Autodesk Fusion 360 part; units mm, degrees
sketch "Sketch1" plane through (0, 0, 0) normal (0, 0, 1) x (1, 0, 0)
  line L0 (0, -25) -> (-80, 0)
  line L1 (-80, 0) -> (0, 25)
  line L2 (80, 0) -> (0, 25)
  line L3 (80, 0) -> (0, -25)
extrude "Extrude1" add sketch "Sketch1" along normal blind 10 makes body 1
fillet "Fillet3" radius 20 1 edges at (0, 25, 5) on bodies 1
fillet "Fillet4" radius 20 1 edges at (0, -25, 5) on bodies 1
sketch "Sketch5" plane through (0, 0, 10) normal (0, 0, 1) x (-1, 0, 0)
  arc A0 (5.9655, 23.1358) -> (-5.9655, 23.1358) centre (0, 4.0462) ccw
  line L0 (-5.9655, 23.1358) -> (-80, 0)
  line L1 (-80, 0) -> (-5.9655, -23.1358)
  arc A1 (-5.9655, -23.1358) -> (5.9655, -23.1358) centre (0, -4.0462) ccw
  line L2 (5.9655, -23.1358) -> (80, 0)
  line L3 (80, 0) -> (5.9655, 23.1358)
  circle A2 centre (0, 0) radius 20
  circle A3 centre (0, 0) radius 12.5
  dimension "d19" = 25
extrude "Extrude5" add sketch "Sketch5" along normal blind 25 contours A2 bodies 1
extrude "Extrude6" cut 1 faces at (-0.8448, -2.1525, 10) along direction (0, 0, -1) blind 60 on bodies 1 bodies 1
sketch "Sketch8" plane through (0, 0, 0) normal (0, 1, 0) x (1, 0, 0)
  line L0 (-20, -30) -> (-30, -10)
  line L1 (-30, -10) -> (-20, -10)
  line L2 (-20, -10) -> (-20, -30)
  line L3 (20, -30) -> (30, -10)
  line L4 (30, -10) -> (20, -10)
  line L5 (20, -10) -> (20, -30)
extrude "Extrude8" add sketch "Sketch8" along normal blind 2.5 separate body makes body 2 at (-23.3333, 0, 16.6667) makes body 3 at (23.3333, 0, 16.6667)
extrude "Extrude9" add 1 faces at (-23.3333, 0, 16.6667) along direction (0, -1, 0) blind 2.5 on bodies 2 bodies 2 3 1
extrude "Extrude10" add 1 faces at (23.3333, 0, 16.6667) along direction (0, -1, 0) blind 2.5 on bodies 3 bodies 3 2
fillet "Fillet5" radius 5 1 edges at (-80, 0, 5) on bodies 3
fillet "Fillet6" radius 5 1 edges at (80, 0, 5) on bodies 3
sketch "Sketch9" plane through (0, 0, 10) normal (0, 0, 1) x (-1, 0, 0)
  arc A0 (-20, 0) -> (20, 0) centre (0, 0) ccw
  line L0 (-20, 0) -> (-20, -2.5)
  line L1 (-20, -2.5) -> (-30, -2.5)
  line L2 (-30, -2.5) -> (-30, 2.5)
  line L3 (-30, 2.5) -> (-20, 2.5)
  line L4 (-20, 2.5) -> (-20, 0)
  arc A1 (20, 0) -> (-20, 0) centre (0, 0) ccw
  line L5 (20, 0) -> (20, 2.5)
  line L6 (20, 2.5) -> (30, 2.5)
  line L7 (30, 2.5) -> (30, -2.5)
  line L8 (30, -2.5) -> (20, -2.5)
  line L9 (20, -2.5) -> (20, 0)
  arc A2 (-64.7283, 4.7724) -> (-64.7283, -4.7724) centre (-63.2369, 0) ccw
  line L10 (-64.7283, -4.7724) -> (-5.9655, -23.1358)
  arc A3 (-5.9655, -23.1358) -> (5.9655, -23.1358) centre (0, -4.0462) ccw
  line L11 (5.9655, -23.1358) -> (64.7283, -4.7724)
  arc A4 (64.7283, -4.7724) -> (64.7283, 4.7724) centre (63.2369, 0) ccw
  line L12 (64.7283, 4.7724) -> (5.9655, 23.1358)
  arc A5 (5.9655, 23.1358) -> (-5.9655, 23.1358) centre (0, 4.0462) ccw
  line L13 (-5.9655, 23.1358) -> (-64.7283, 4.7724)
  circle A6 centre (60, 0) radius 4
  circle A7 centre (-60, 0) radius 4
  dimension "d34" = 8
  dimension "d35" = 8
extrude "Extrude11" cut sketch "Sketch9" against normal blind 40 contours A6 | A7 bodies 3
CAD build for the part. Positions are in the model's coordinates, mm. A direction names the side the tool comes from. Coordinates: 2 decimals unless noted, no trailing zeros. Order: outer loops, then holes, each group sorted by start corner. A loop starts at its lowest first (then second) coordinate and runs counter-clockwise, first axis right, second up.
Item 1: Two-plate mould, pull along Y, no slides. Class faces 4 (the face through (35.758, 13.826, 4.93)), 5 (the face through (14, 0, 0)), 6 (the face through (-63.815, -1.201, 5.07)): +Y half, -Y half, draft (parallel to the pull), parting line (faces both ways), or undercut.
Check sheet entries:
face 4: +Y half
face 5: draft
face 6: undercut
Item 2: Band-saw the part on D-D on x = -28. List the corners of the cut face in (y, z), plus the area to 3 significant figures.
Check sheet entries:
outline: (-16.25, 0) - (16.25, 0) - (16.25, 10) - (2.5, 10) - (2.5, 14) - (-2.5, 14) - (-2.5, 10) - (-16.25, 10) - close
area: 345 mm2
Item 3: Band-saw the part on C-C on y = -11. List the corners of the cut face in (x, z).
Check sheet entries:
outline: (-44.8, 0) - (-5.94, 0) - (-5.94, 35) - (-16.7, 35) - (-16.7, 10) - (-44.8, 10) - close; (5.94, 0) - (44.8, 0) - (44.8, 10) - (16.7, 10) - (16.7, 35) - (5.94, 35) - close
Item 4: Band-saw the part on B-B on x = -60. List the corners of the cut face in (y, z), plus the area to 3 significant figures.
Check sheet entries:
outline: (-6.25, 0) - (-4, 0) - (-4, 10) - (-6.25, 10) - close; (4, 0) - (6.25, 0) - (6.25, 10) - (4, 10) - close
area: 45.0 mm2
Item 5: Drill centre lines: L1, parallel to X at y = 0, z = 5.25; L2, parallel to Y at x = 0, z = 13; L3, parallel to Y at x = 60, z = 4. Where is each one in solid material? Low to high.
Check sheet entries:
L1: x = -68.24 to -64, -56 to -12.5, 12.5 to 56, 64 to 68.24
L2: y = -20 to -12.5, 12.5 to 20
L3: y = -6.25 to -4, 4 to 6.25
Item 6: 3-axis set-ups, long thin cutter, end or side, ignore diameter. For faces 1 (the face through (24, 2.5, 18)), 2 (the face through (24, -2.5, 18)), 3 (the face through (-23, 2.5, 15)): which of +Z, -Z, +X, -X, +Y, -Y reach the whole face in a straight line?
Check sheet entries:
face 1: +Z, +X, +Y
face 2: +Z, +X, -Y
face 3: +Z, -X, +Y
Item 7: Pin check, flat tips, straight feed: pin 1 Ø4 at (y, z) = (1, 20) entering from -X; pin 2 Ø6 at (x, y) = (-53, -8) entering from +Z; pin 3 Ø8 at (y, z) = (-18.5, 17.5) entering from -X (3 decimals); pin 4 Ø5 at (x, z) = (-27, 23.5) entering from -Y. Stop position of each tip, or through.
Check sheet entries:
pin 1: stops at x = -26
pin 2: stops at z = 10
pin 3: stops at x = -13.775
pin 4: passes through
